Verification items for the finished model (mm, model axes). Coordinates: 2 decimals unless noted, no trailing zeros. Order: outer loops, then holes, each group sorted by start corner. A loop starts at its lowest first (then second) coordinate and runs counter-clockwise, first axis right, second up. Notation, with made-up numbers: M 21,-11 L 50,-11 A13 ccw 50,0 Z; hole C -38.75,60 d7. An arc over 180 degrees is marked long. Return JSON: item names as keys, results as strings. Group by question number.
Q1. Section check B-B, the plane z = 0. Enter the section's corners in (x, y).
Q2. Section check D-D, the plane z = 26.5. Enter the section's corners in (x, y).
Q3. Go/stop test with flat-tipped pins: pin 1 Ø1 at (y, z) = (1.5, 28) entering from +X; pin 2 Ø1 at (x, y) = (-1.5, 1.5) entering from +Z; pin 3 Ø1 at (y, z) = (0.5, -5) entering from +X. Record where each tip stops, or that it passes through.
Q4. Thickness scan on probe 1 along X at (y, z) = (1.1, -0.5); probe 2 along X at (y, z) = (1.1, 6.5); probe 3 along Z at (x, y) = (3, 1.1). Record the ranges inside material, lowest first.
Q5. Section check C-C, the plane y = 1.55. Enter the section's corners in (x, z).
Q6. Section check A-A, the plane x = 0. Enter the section's corners in (y, z), then the cut area to 3 significant figures.
Autodesk Inventor part; units mm, degrees
ref_plane "YZ Plane" through (0, 0, 0) normal (1, 0, 0) x (0, 1, 0)
ref_plane "XZ Plane" through (0, 0, 0) normal (0, 1, 0) x (-1, 0, 0)
ref_plane "XY Plane" through (0, 0, 0) normal (0, 0, 1) x (1, 0, 0)
sketch "Sketch1" plane through (0, 0, 0) normal (0, 1, 0) x (-1, 0, 0)
  circle A0 centre (0, 0) radius 41
  line L0 (-4, 10) -> (4, 10)
  line L1 (4, 10) -> (4, -10)
  line L2 (4, -10) -> (-4, -10)
  line L3 (-4, -10) -> (-4, 10)
  line L4 (-4, 10) -> (4, -10) construction
  line L5 (4, 10) -> (-4, -10) construction
  circle A1 centre (0, 0) radius 27.3333 construction
  line L6 (0, 20.8333) -> (0, 33.8333) construction
  line L7 (4, 29.8333) -> (4, 24.8333)
  line L8 (-4, 29.8333) -> (-4, 24.8333)
  arc A2 (2.7505, 27.1946) -> (2.625, 27.3333) centre (0, 24.8333) ccw
  arc A3 (-2.625, 27.3333) -> (-2.7505, 27.1946) centre (0, 24.8333) ccw
  arc A4 (-4, 24.8333) -> (4, 24.8333) centre (0, 24.8333) ccw
  arc A5 (2.51, 27.2178) -> (2.625, 27.3333) centre (0, 29.8333) ccw
  arc A6 (4, 29.8333) -> (-4, 29.8333) centre (0, 29.8333) ccw
  arc A7 (-2.625, 27.3333) -> (-2.51, 27.2178) centre (0, 29.8333) ccw
  point P0 (0, 27.3333)
  point P1 (1.5875, 22.7958)
  dimension "d0" = 8
  dimension "d1" = 20
  dimension "d2" = 82
  dimension "d4" = 54.6667
  dimension "d5" = 13
  dimension "d11" = 4
extrude "Extrusion1" add sketch "Sketch1" along normal blind 2
properties part number "Tic-Tac Baseplate v2"
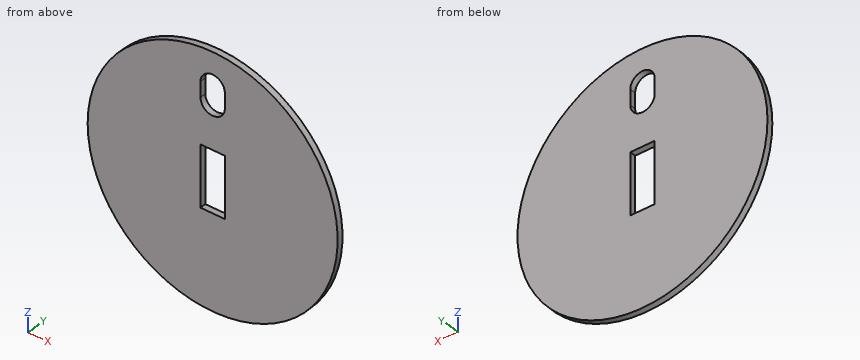
Numbers:
{
 "1": {"outline": "M -41,0 L -4,0 L -4,2 L -41,2 Z; M 4,0 L 41,0 L 41,2 L 4,2 Z"},
 "2": {"outline": "M -31.28,0 L -4,0 L -4,2 L -31.28,2 Z; M 4,0 L 31.28,0 L 31.28,2 L 4,2 Z"},
 "3": {"pin 1": "stops at x = 30.41", "pin 2": "stops at z = 40.99", "pin 3": "stops at x = 40.75"},
 "4": {"probe 1": "x = -41 to -4, 4 to 41", "probe 2": "x = -40.48 to -4, 4 to 40.48", "probe 3": "z = -40.89 to -10, 10 to 22.19, 32.48 to 40.89"},
 "5": {"outline": "C 0,0 d82; hole M -4,-10 L 4,-10 L 4,10 L -4,10 Z; hole M -4,24.83 A4 ccw 4,24.83 L 4,29.83 A4 ccw -4,29.83 Z"},
 "6": {"outline": "M 0,-41 L 2,-41 L 2,-10 L 0,-10 Z; M 0,10 L 2,10 L 2,20.83 L 0,20.83 Z; M 0,33.83 L 2,33.83 L 2,41 L 0,41 Z", "area": "98.0 mm2"}
}
